Geometry: final body of the model. Coordinates: model frame, mm. A direction names the side the tool comes from. Give positions to 0.01 mm unless a question says otherwise; leave off trailing zeros. Write each loop counter-clockwise with the first axis right and the second up, starting at its lowest first coordinate (ties: lowest second). Pieces come first, ordered by that corner, then holes.
Q1. Line query: L1, parallel to X at y = 16, z = 0.35; L2, parallel to Z at x = 48.5, y = 13; L3, parallel to Y at x = -28, z = 1.9. Output: solid intervals per line, ascending.
Q2. Draft query along X for faces 1 (the face through (-55.39, 0.43, 2.1)), 2 (the face through (-1, 0, 4)), 3 (the face through (-56.109, 0.434, 2.797)), 4 (the face through (55.39, 0.43, 2.1)). Return one class per face: pulls with the +X half, pulls with the -X half, needs draft (parallel to the pull), parting line crosses it, or undercut.
Q3. Pin query (flat end, axial travel): pin 1 (5 mm diameter, centred on x = -11.5, y = -4.5, fed in from -Z); pin 2 (2 mm diameter, centred on x = -18, z = 2, fed in from +Y). Return the tip coordinate at first contact, or that it passes through.
Q4. Cut plane A-A on y = 0. Count the separate pieces of the cut face and the enclosed holes in it, plus the area to 3 significant figures.
Q5. Reachability of faces 5 (the face through (0.75, 33.14, 2.1)), 6 (the face through (0.746, -33.859, 2.797)) from +Z, -Z, +X, -X, +Y, -Y: full face, straight path, thin tool, end or side. Return the list, or none.
Q6. Cut plane C-C on z = 1.95. Return the cut outline in (x, y).
```python
from build123d import *

# Parameters (mm, degrees)
F0_W           = 114.5
F0_H           = 70
F1_DEPTH       = 4
F2_R           = 3.99999
F3_T           = -1
F5_D           = 2
F5_CSINK_D     = 4
F5_CSINK_ANGLE = 90


# Not quite as in the source:
# - a fillet or chamfer is up to 0.001 mm smaller than in the source, because OpenCascade refuses the exact size


with BuildPart() as f1:
    # F0 (on Top) → F1 (new body)
    with BuildSketch(Plane.XY):
        Rectangle(F0_W, F0_H)
    extrude(amount=F1_DEPTH)

    # F2 (radius 4 in the source; OpenCascade refuses exactly that, so slightly less here)
    f2_edges = [f1.edges().sort_by_distance(p)[0] for p in [
        (-57.25, 0, 4),
        (0, 35, 4),
        (0, -35, 4),
        (-57.25, -35, 2),
        (-57.25, 35, 2),
        (57.25, 35, 2),
        (57.25, 0, 4),
        (57.25, -35, 2),
    ]]
    fillet(f2_edges, radius=F2_R)

    # F3
    f3_openings = [f1.faces().sort_by_distance(p)[0] for p in [
        (0, 0, 0),
    ]]
    offset(amount=F3_T, openings=f3_openings)

    # F5 (through all)
    with Locations(Plane.XY.offset(4)):
        with Locations((41.5, 0), (-41.5, 0)):
            CounterSinkHole(F5_D / 2, F5_CSINK_D / 2, counter_sink_angle=F5_CSINK_ANGLE)


solid = f1.part
```
Data:
1. L1: x = -57.23 to -56.23, 56.23 to 57.23
1. L2: z = 3 to 4
1. L3: y = -34.52 to -33.32, 33.32 to 34.52
2. face 1: undercut
2. face 2: needs draft
2. face 3: pulls with the -X half
2. face 4: undercut
3. pin 1: stops at z = 3
3. pin 2: stops at y = 34.87
4. separate pieces: 3
4. enclosed holes: 0
4. area: 111 mm2
5. face 5: -Z
5. face 6: +Z, +X, -X, -Y
6. outline: (-56.74, -31) arc R3.49 ccw to (-53.25, -34.49) - (53.25, -34.49) arc R3.49 ccw to (56.74, -31) - (56.74, 31) arc R3.49 ccw to (53.25, 34.49) - (-53.25, 34.49) arc R3.49 ccw to (-56.74, 31) - close; hole (-55.53, -31) arc R2.28 ccw to (-53.25, -33.28) - (53.25, -33.28) arc R2.28 ccw to (55.53, -31) - (55.53, 31) arc R2.28 ccw to (53.25, 33.28) - (-53.25, 33.28) arc R2.28 ccw to (-55.53, 31) - close
